Check sheet for the modelled part. Datum: model origin and axes. Units: mm. A direction names the side the tool comes from. Round coordinates to 2 decimals unless told otherwise and drop trailing zeros. Loops run counter-clockwise (first coordinate to the right, second up) from the corner with the lowest first, then second, coordinate; pieces in that order, holes last. Notation, with made-up numbers: M 13,51.25 L 66,51.25 A16 ccw 66,58.25 Z; hole C 60,-8 d11. An arc over 180 degrees is marked long. Write item = value, one per line. Start each with the question number.
(1) Mould release check, pull along Z, two halves, no side actions. Record for faces 4 (the face through (-59.9, 10, 11.6)), 5 (the face through (-67.66, -12.5, 20.46)), 6 (the face through (-1, 6, 23)): pulls with the +Z half, pulls with the -Z half, needs draft (parallel to the pull), parting line crosses it, or undercut.
(2) Cross-section at A-A on z = 11.5. Record the boundary of the cut face in (x, y).
(3) Cross-section at B-B on x = -67.5. Record the boundary of the cut face in (y, z), plus the area to 3 significant figures.
(4) Go/stop test with flat-tipped pins: P1, Ø4.5, axis at x = 67.5, y = -5, coming from the -Z side; P2, Ø8, axis at x = -29, z = 17.5, coming from the -Y side; P3, Ø10.5, axis at x = 14, z = 12.5, coming from the -Y side; P4, Ø3, axis at y = -7.5, z = 3.5, coming from the +X side. Record where each tip stops, or that it passes through.
(5) Set-up check for faces 1 (the face through (0, 5, 5)), 2 (the face through (58.53, 1.1, 20.46)), 3 (the face through (64.9, -4.9, 2.5)): record each of +Z, -Z, +X, -X, +Y, -Y from which the full face is reachable in a straight line by a thin tool's end or side.
(6) Cross-section at C-C on y = -10.75. Record the boundary of the cut face in (x, z).
(7) Scan lines: L1, parallel to Y at x = -67.5, z = 21.65; L2, parallel to Z at x = -45, y = 6.5; L3, parallel to X at y = -5, z = 19. Record each from-to range of solid material in increasing order. Write a range as from..to.
(8) Cross-section at D-D on x = 33. Record the boundary of the cut face in (y, z).
from build123d import *

# Parameters (mm, degrees)
F0_R     = 2.6
F1_DEPTH = 23
F2_W     = 12.5
F2_H     = 13
F2_W_2   = 16.9316109251
F3_DEPTH = 150.001
F4_R     = 2.6
F5_DEPTH = 25.001


with BuildPart() as f1:
    # F0 (on Top) → F1 (new body)
    with BuildSketch(Plane.XY):
        with BuildLine():
            Line((75, -5), (75, 12.5))
            Line((75, 12.5), (-75, 12.5))
            Line((-75, 12.5), (-75, -5))
            ThreePointArc((-75, -5), (-67.5, -12.5), (-60, -5))
            Line((-60, -5), (-60, -2.4001719305))
            ThreePointArc((-60, -2.4001719305), (-58.5647992072, 1.0646753177), (-55.0999320596, 2.499828069))
            Line((-55.0999320596, 2.499828069), (55.1000685735, 2.4983001034))
            ThreePointArc((55.1000685735, 2.4983001034), (58.5648478814, 1.0630993111), (60.0000006331, -2.4016998961))
            Line((60.0000006331, -2.4016998961), (60.0000006331, -4.9969182812))
            ThreePointArc((60.0000006331, -4.9969182812), (67.4984591406, -12.4999998417), (75, -5))
        make_face()
        with Locations((-67.5, -5)):
            Circle(F0_R, mode=Mode.SUBTRACT)
        with Locations((67.5, -5)):
            Circle(F0_R, mode=Mode.SUBTRACT)
    extrude(amount=F1_DEPTH)

    # F2 (on face) → F3 (cut, through all)
    with BuildSketch(Plane(origin=(-75, 0, 0), x_dir=(0, -1, 0), z_dir=(-1, 0, 0))):
        with Locations((-1.25, 11.5)):
            Rectangle(F2_W, F2_H)
        with Locations((13.4658054625, 11.5)):
            Rectangle(F2_W_2, F2_H)
    extrude(amount=-F3_DEPTH, mode=Mode.SUBTRACT)

    # F4 (on face) → F5 (cut, through all)
    with BuildSketch(Plane(origin=(0, 12.5, 0), x_dir=(-1, 0, 0), z_dir=(0, 1, 0))):
        with Locations((62.5, 11.5)):
            Circle(F4_R)
        with Locations((-62.5, 11.5)):
            Circle(F4_R)
    extrude(amount=-F5_DEPTH, mode=Mode.SUBTRACT)


solid = f1.part
Result:
q1.face_4 = undercut
q1.face_5 = needs draft
q1.face_6 = pulls with the +Z half
q2.outline = M -75,7.5 L -65.1,7.5 L -65.1,12.5 L -75,12.5 Z; M -59.9,7.5 L 59.9,7.5 L 59.9,12.5 L -59.9,12.5 Z; M 65.1,7.5 L 75,7.5 L 75,12.5 L 65.1,12.5 Z
q3.outline = M -12.5,0 L -7.6,0 L -7.6,5 L -12.5,5 Z; M -12.5,18 L -7.6,18 L -7.6,23 L -12.5,23 Z; M -2.4,0 L 12.5,0 L 12.5,23 L -2.4,23 L -2.4,18 L 7.5,18 L 7.5,5 L -2.4,5 Z
q3.area = 263 mm^2
q4.P1 = through
q4.P2 = 2.5
q4.P3 = 7.5
q4.P4 = 74.93
q5.face_1 = +X, -X, -Y
q5.face_2 = +Z, -Z, -Y
q5.face_3 = +Z, -Z
q6.outline = M -72.32,0 L -62.68,0 L -62.68,5 L -72.32,5 Z; M -72.32,18 L -62.68,18 L -62.68,23 L -72.32,23 Z; M 62.68,0 L 72.32,0 L 72.32,5 L 62.68,5 Z; M 62.68,18 L 72.32,18 L 72.32,23 L 62.68,23 Z
q7.L1 = -12.5..-7.6, -2.4..12.5
q7.L2 = 0..5, 18..23
q7.L3 = -75..-70.1, -64.9..-60, 60..64.9, 70.1..75
q8.outline = M 2.5,0 L 12.5,0 L 12.5,23 L 2.5,23 L 2.5,18 L 7.5,18 L 7.5,5 L 2.5,5 Z
